Geometry: final body of the model. Coordinates: model frame, mm. Face numbers are marked on the shaded views. A direction names the side the tool comes from. Give positions to 0.01 mm unless a question says otherwise; leave off trailing zeros. Write each loop counter-clockwise with the first axis right and the second up, starting at its lowest first coordinate (ties: lowest second). Pieces come first, ordered by that corner, then holes. Notation, with made-up numbers: (-14.75, -29.75) -> (20.25, -29.75) arc R23 cw to (20.25, -20.75) -> close; hole circle Ø6 at (81, 82). An arc over 180 degrees is marked (long way). Answer as a JSON object with one key per item and string values.
from build123d import *

# Parameters (mm, degrees)
F0_W     = 17.8
F0_H     = 17.8
F1_DEPTH = 5
F2_R     = 4
F3_T     = -1


with BuildPart() as f1:
    # F0 (on Top) → F1 (new body)
    with BuildSketch(Plane.XY):
        with Locations((-8.9, 8.9)):
            Rectangle(F0_W, F0_H)
    extrude(amount=F1_DEPTH)

    # F2
    f2_edges = [f1.edges().sort_by_distance(p)[0] for p in [
        (0, 8.9, 5),
    ]]
    fillet(f2_edges, radius=F2_R)

    # F3
    f3_openings = [f1.faces().sort_by_distance(p)[0] for p in [
        (-8.9, 8.9, 0),
        (-17.8, 8.9, 2.5),
    ]]
    offset(amount=F3_T, openings=f3_openings)


solid = f1.part
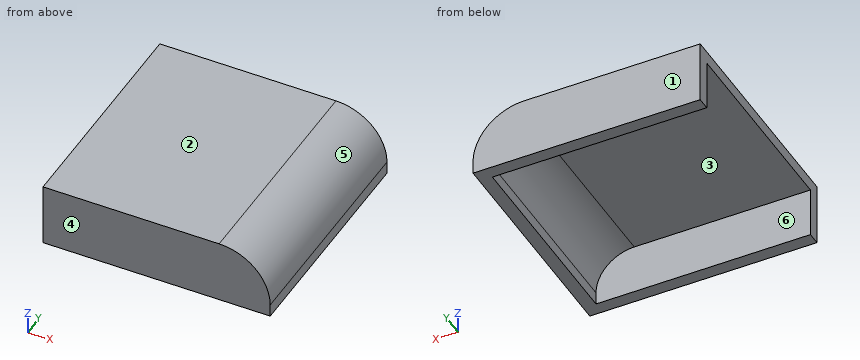
Q1. Set-up query: the marked faces 5 and 6. Return all of +Z, -Z, +X, -X, +Y, -Y with unobstructed straight access to the full face (end or side cutting, diameter ignored); none if empty.
Values:
{"face 5": "+Z, +X, +Y, -Y", "face 6": "-Z, -X"}
Q2. Mould query, pull axis Y, two halves, no side actions, for the marked faces 1, 2, 3 and 4. Classes: pulls with the +Y half, pulls with the -Y half, needs draft (parallel to the pull), parting line crosses it, or undercut.
Values:
{"face 1": "pulls with the +Y half", "face 2": "needs draft", "face 3": "undercut", "face 4": "pulls with the -Y half"}
Q3. First-contact query: P1, Ø0.8, axis at y = 6.5, z = 0.5, coming from the -X side; P2, Ø5, axis at x = -4, y = 4, coming from the -Z side. Flat tips, straight axial feed; report the tip coordinate or a pass-through.
Values:
{"P1": "x = -1", "P2": "z = 2.66"}
Q4. Cut plane B-B (z = 0.4). Return the cut outline in (x, y), and give its area (3 significant figures).
Values:
{"outline": "(-17.8, 0) -> (0, 0) -> (0, 17.8) -> (-17.8, 17.8) -> (-17.8, 16.8) -> (-1, 16.8) -> (-1, 1) -> (-17.8, 1) -> close", "area": "51.4 mm²"}
Q5. Cut plane A-A (x = -7.5). Return the cut outline in (y, z), and give its area (3 significant figures).
Values:
{"outline": "(0, 0) -> (1, 0) -> (1, 4) -> (16.8, 4) -> (16.8, 0) -> (17.8, 0) -> (17.8, 5) -> (0, 5) -> close", "area": "25.8 mm²"}
Q6. Material intervals for L1, parallel to Y at x = -2.25, z = 1.95; L2, parallel to Z at x = -14.5, y = 4; L3, parallel to X at y = 3.25, z = 3.55, sorted ascending. Write a range as from..to.
Values:
{"L1": "0..1, 16.8..17.8", "L2": "4..5", "L3": "-2.42..-0.92"}
